Read the model definition and answer for the solid it produces. Units are mm, in the model's axes. Face numbers are marked on the shaded views. A direction names the side the tool comes from. Give positions to 0.01 mm unless a question says otherwise; leave off trailing zeros. Write each loop counter-clockwise with the first axis right and the second up, starting at its lowest first coordinate (ties: lowest second). Pieces come first, ordered by that corner, then holes. Notation, with made-up numbers: (-3.5, 37) -> (47.5, 37) arc R20 ccw to (47.5, 66) -> close; hole circle Ø8 at (82.25, 77.5). An arc over 180 degrees is marked (long way). Put each result on its own line as item: value. Start each with the question number.
from build123d import *

# Parameters (mm, degrees)
SKETCH2_R           = 13.5
SKETCH2_R_2         = 2.65
BOSS_EXTRUDE1_DEPTH = 8
BOSS_EXTRUDE2_DEPTH = 8
CIRPATTERN1_COUNT   = 28
SKETCH3_R           = 11
CUT_EXTRUDE1_DEPTH  = 1
SKETCH4_R           = 1.1
CUT_EXTRUDE2_DEPTH  = 24.010866998


with BuildPart() as part:
    # Sketch2 → Boss-Extrude1 (new body)
    with BuildSketch(Plane.XY):
        Circle(SKETCH2_R)
        Circle(SKETCH2_R_2, mode=Mode.SUBTRACT)
    extrude(amount=BOSS_EXTRUDE1_DEPTH)

    # Sketch2_3 → Boss-Extrude2 (add)
    with BuildSketch(Plane.XY):
        with BuildLine():
            ThreePointArc((1, 13.462912018), (0.799796473, 14.532930237), (0.3, 15.5))
            Line((0.3, 15.5), (-0.3, 15.5))
            ThreePointArc((-0.3, 15.5), (-0.799796473, 14.532930237), (-1, 13.462912018))
            ThreePointArc((-1, 13.462912018), (0, 13.5), (1, 13.462912018))
        make_face()
    boss_extrude2 = extrude(amount=BOSS_EXTRUDE2_DEPTH)

    # CirPattern1: Boss-Extrude2 ×28 about axis
    cirpattern1_axis = Axis((0, 0, 0), (0, 0, 1))
    for i in range(1, CIRPATTERN1_COUNT):
        add(boss_extrude2.rotate(cirpattern1_axis, i * 360 / CIRPATTERN1_COUNT))

    # Sketch3 → Cut-Extrude1 (cut)
    with BuildSketch(Plane.XY.offset(8)):
        Circle(SKETCH3_R)
    extrude(amount=-CUT_EXTRUDE1_DEPTH, mode=Mode.SUBTRACT)

    # Sketch4 → Cut-Extrude2 (cut, through all)
    with BuildSketch(Plane.XY.offset(7)):
        with Locations((-7, 0)):
            Circle(SKETCH4_R)
        with Locations((7, 0)):
            Circle(SKETCH4_R)
    extrude(amount=-CUT_EXTRUDE2_DEPTH, mode=Mode.SUBTRACT)


solid = part.part
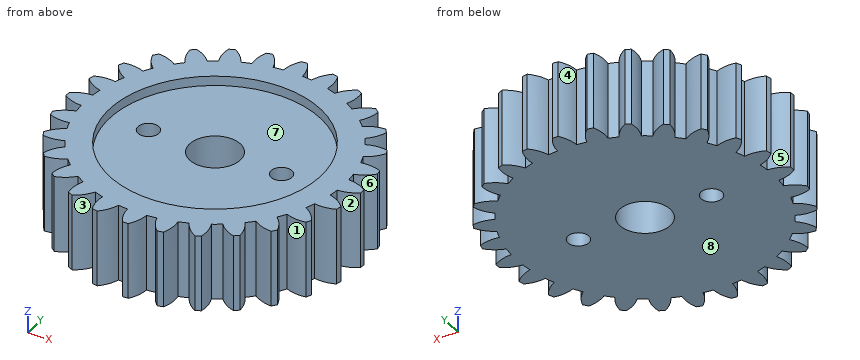
1) For the marked faces 1, 2, 3, 4 and 5, determine the directions among +Z, -Z, +X, -X, +Y, -Y from which every point of the face is accessible in a straight line to the end or side of a thin tool.
2) Each of these flat-tipped pins is pushed along its axis until it touches: pin 1 Ø1.5 at (x, z) = (11, 7) entering from +Y; pin 2 Ø3 at (x, z) = (-2.5, 7) entering from -Y; pin 3 Ø2.5 at (x, y) = (-7, 0) entering from +Z. Where does it stop, or does it pass through?
3) Straight lines are drawn through the part: line 1 (X direction, y = -12, z = 3.5); line 2 (Y direction, x = 0, z = 4.5). For each, find the intervals that lie inside material, in ascending order. Write a range as [from, to].
4) A cutting plane is placed at B-B on y = 5.5. Give the vertices of the cut face in (x, z).
5) A cutting plane is placed at A-A on z = 6.5. State how many separate pieces and enclosed holes the cut face has, and give its area (3 significant figures).
6) For a pull along X with two mould halves and no side action, classify the marked faces 6, 7 and 8 as pulls with the +X half, pulls with the -X half, needs draft (parallel to the pull), parting line crosses it, or undercut.
Results found:
1. face 1: +Z, -Z
1. face 2: +Z, -Z, +X
1. face 3: +Z, -Z, -Y
1. face 4: +Z, -Z, +Y
1. face 5: +Z, -Z, -X
2. pin 1: stops at y = 9.89
2. pin 2: stops at y = -15.18
2. pin 3: stops at z = 7
3. line 1: x = [-9.81, -8.67], [-6.86, 6.86], [8.67, 9.81]
3. line 2: y = [-15.5, -2.65], [2.65, 15.5]
4. outline: (-13.35, 0) -> (13.35, 0) -> (13.35, 8) -> (9.53, 8) -> (9.53, 7) -> (-9.53, 7) -> (-9.53, 8) -> (-13.35, 8) -> close
5. separate pieces: 1
5. enclosed holes: 3
5. area: 628 mm²
6. face 6: pulls with the +X half
6. face 7: undercut
6. face 8: needs draft
